```python
from build123d import *

# Parameters (mm, degrees)
SKETCH1_W           = 5
SKETCH1_H           = 98.8
SKETCH1_H_2         = 16.000962119
BOSS_EXTRUDE1_DEPTH = 5


with BuildPart() as part:
    # Sketch1 → Boss-Extrude1 (new body)
    with BuildSketch(Plane(origin=(0, 0, 0), x_dir=(1, 0, 0), z_dir=(0, 1, 0))):
        Polygon((-280, 247), (-180.213569057, 247), (-180.213569057, 242), (-164.213569057, 242), (-164.213569057, 247), (-148.213569057, 247), (-148.213569057, 242), (-132.213569057, 242), (-132.213569057, 247), (-116.213569057, 247), (-116.213569057, 242), (-100.213569057, 242), (-100.213569057, 247), (99.786430943, 247), (99.786430943, 242), (115.786430943, 242), (115.786430943, 247), (131.786430943, 247), (131.786430943, 242), (147.786430943, 242), (147.786430943, 247), (163.786430943, 247), (163.786430943, 242), (179.786430943, 242), (179.786430943, 247), (280, 247), (280, -247), (-280, -247), align=None)
        with Locations((-217.5, -98.8)):
            Rectangle(SKETCH1_W, SKETCH1_H, mode=Mode.SUBTRACT)
        with Locations((217.5, -98.8)):
            Rectangle(SKETCH1_W, SKETCH1_H, mode=Mode.SUBTRACT)
        with Locations((-202.5, -82.801443178)):
            Rectangle(SKETCH1_W, SKETCH1_H_2, mode=Mode.SUBTRACT)
        with Locations((217.5, 98.8)):
            Rectangle(SKETCH1_W, SKETCH1_H, mode=Mode.SUBTRACT)
        with Locations((-217.5, 98.8)):
            Rectangle(SKETCH1_W, SKETCH1_H, mode=Mode.SUBTRACT)
        with Locations((202.5, -114.803367415)):
            Rectangle(SKETCH1_W, SKETCH1_H_2, mode=Mode.SUBTRACT)
        with Locations((202.5, -82.801443178)):
            Rectangle(SKETCH1_W, SKETCH1_H_2, mode=Mode.SUBTRACT)
        with Locations((-202.5, -114.803367415)):
            Rectangle(SKETCH1_W, SKETCH1_H_2, mode=Mode.SUBTRACT)
    extrude(amount=BOSS_EXTRUDE1_DEPTH)


solid = part.part
```
The listing builds one solid part. Answer for the finished solid, in the listing's coordinates (mm). Coordinates: 2 decimals unless noted, no trailing zeros. Loops run counter-clockwise (first coordinate to the right, second up) from the corner with the lowest first, then second, coordinate; pieces in that order, holes last. Notation, with made-up numbers: M 26.5,-37.75 L 61.5,-37.75 A17 ccw 61.5,-33.75 Z; hole C 75.5,74.25 d4. An arc over 180 degrees is marked long. Answer as a JSON object with one key per item and string values. Group by question number.
Item 1: This flat-tipped pin is pushed along its axis until it touches: P1, Ø2.5, axis at x = -172, y = 3, coming from the -Z side. Where does it stop, or does it pass through?
Item 2: Consider L1, parallel to X at y = 3, z = -85; L2, parallel to X at y = 3.45, z = 78; L3, parallel to Z at x = -146, y = 4.4. Determine where each line is inside the solid, lowest interval first.
Item 3: Section A-A (z = 59.5) is taken. Write down the section's boundary in (x, y), and give its area (3 significant figures).
Solved:
{
 "1": {"P1": "stops at z = -242"},
 "2": {"L1": "x = -280 to -220, -215 to 215, 220 to 280", "L2": "x = -280 to -220, -215 to -205, -200 to 200, 205 to 215, 220 to 280", "L3": "z = -242 to 247"},
 "3": {"outline": "M -280,0 L -220,0 L -220,5 L -280,5 Z; M -215,0 L 215,0 L 215,5 L -215,5 Z; M 220,0 L 280,0 L 280,5 L 220,5 Z", "area": "2,750 mm2"}
}
